Geometry: final body of the model. Coordinates: model frame, mm. A direction names the side the tool comes from. Coordinates: 2 decimals unless noted, no trailing zeros. Order: outer loops, then holes, each group sorted by start corner. A loop starts at its lowest first (then second) coordinate and runs counter-clockwise, first axis right, second up. Notation, with made-up numbers: M -34.5,-10 L 0.5,-10 A37 ccw 0.5,26 Z; hole C 39,41 d10. An arc over 180 degrees is marked long. Use CSV: the item, a comma, the result in double quotes. Start each with the question number.
Q1. Section query A-A, the plane z = -116.5. Output: boundary loops of the cut face in (x, y).
Q2. Access query for faces 1 (the face through (7, 5.5, -150)), 2 (the face through (2, 6, -127.5)), 3 (the face through (2, 4, -142.5)), 4 (the face through (3.5, 6.883, 151.232)). Directions: +Z, -Z, +X, -X, +Y, -Y. A direction counts if a zero-diameter tool reaches every point of the face in a straight line with its end or side. Return the directions, or none.
Q3. First-contact query: P1, Ø5, axis at y = 2, z = 48.5, coming from the +X side; P2, Ø2, axis at y = 2, z = -70.5, coming from the -X side; P3, Ø5, axis at x = 3, z = -82, coming from the +Y side. Flat tips, straight axial feed; report the tip coordinate or a pass-through.
Q4. Mould query, pull axis X, two halves, no side actions, for faces 5 (the face through (2.168, 8.497, -151.486)), 6 (the face through (4, 6, -146)), 7 (the face through (-3.5, 5, -139)), 8 (the face through (7.2, 5.1, 150)). Classes: +X half, -X half, draft (parallel to the pull), parting line (faces both ways), or undercut.
Q5. Ray query, probe 1 along Z at (x, y) = (7.25, 4); probe 2 along Z at (x, y) = (2, 7.7); probe 3 along Z at (x, y) = (2, 1). Return the intervals inside material, ascending.
Autodesk Inventor part; units mm, degrees
ref_plane "YZ Plane" through (0, 0, 0) normal (1, 0, 0) x (0, 1, 0)
ref_plane "XZ Plane" through (0, 0, 0) normal (0, 1, 0) x (-1, 0, 0)
ref_plane "XY Plane" through (0, 0, 0) normal (0, 0, 1) x (1, 0, 0)
sketch "Sketch1" plane through (0, 0, 0) normal (0, 0, 1) x (1, 0, 0)
  line L0 (0, 0) -> (4, 0)
  line L1 (4, 0) -> (4, 4)
  line L2 (4, 4) -> (0, 4)
  line L3 (0, 4) -> (0, 0)
  dimension "d0" = 4
  dimension "d1" = 4
extrude "Extrusion1" add sketch "Sketch1" along normal blind 138.5
sketch "Sketch3" plane through (0, 0, 138.5) normal (0, 0, 1) x (1, 0, 0)
  line L0 (0, 0) -> (4, 0)
  line L1 (-3.5, 0) -> (7.5, 0)
  line L2 (7.5, 0) -> (7.5, 8)
  line L3 (7.5, 8) -> (-3.5, 8)
  line L4 (-3.5, 8) -> (-3.5, 0)
  point P0 (2, 0)
  dimension "d4" = 11
  dimension "d5" = 8
extrude "Extrusion2" add sketch "Sketch3" along normal blind 11.5
sketch "Sketch4" plane through (0, 0, 0) normal (0, -1, 0) x (1, 0, 0)
  line L0 (7.5, 138.5) -> (7.5, 150)
  line L1 (-3.5, 150) -> (7.5, 150)
  line L2 (-1.75, 146) -> (5.75, 146)
  line L3 (5.75, 146) -> (5.75, 142.5)
  line L4 (5.75, 142.5) -> (-1.75, 142.5)
  line L5 (-1.75, 142.5) -> (-1.75, 146)
  point P0 (2, 146)
  point P1 (2, 150)
  point P2 (5.75, 144.25)
  point P3 (7.5, 144.25)
  dimension "d8" = 7.5
  dimension "d9" = 3.5
extrude "Extrusion3" cut sketch "Sketch4" against normal blind 8
sketch "Sketch5" plane through (0, 0, 150) normal (0, 0, 1) x (1, 0, 0)
  circle A0 centre (2, 4) radius 2.1
  point P0 (0, 0)
  dimension "d12" = 4.2
extrude "Extrusion4" cut sketch "Sketch5" against normal up to surface (7.5 mm away)
sketch "Sketch6" plane through (-3.5, 8, 138.5) normal (0, 1, 0) x (1, 0, 0)
  line L0 (11, 0) -> (0, 0)
  line L1 (0, 0) -> (0, -11.5)
  line L2 (11, -11.5) -> (0, -11.5)
  line L3 (11, 0) -> (11, -11.5)
  point P0 (3.5, 138.5)
extrude "Extrusion5" add sketch "Sketch6" along normal blind 1
mirror "Mirror2" about plane through (0, 0, 0) normal (0, 0, 1) of "Extrusion1", "Extrusion5", "Extrusion2", "Extrusion3", "Extrusion4"
sketch "Sketch7" plane through (0, 0, 150) normal (0, 0, 1) x (1, 0, 0)
  line L0 (-3.5, 0) -> (7.5, 0)
  arc A0 (4.0616, 0) -> (-0.0616, 0) centre (2, 4) ccw
  line L1 (0, 0) -> (-0.0616, 0)
  line L2 (-0.0616, 0) -> (4.0616, 0)
  circle A1 centre (2, 4) radius 3.25
  dimension "d17" = 9
  dimension "d18" = 6.5
extrude "Extrusion6" add sketch "Sketch7" along normal blind 2.5
sketch "Sketch8" plane through (-3.5, 8, 138.5) normal (0, -1, 0) x (1, 0, 0)
  line L0 (1.75, 7.5) -> (1.75, 4)
  line L1 (1.75, 4) -> (9.25, 4)
  line L2 (9.25, 4) -> (9.25, 7.5)
  line L3 (9.25, 7.5) -> (1.75, 7.5)
  point P0 (3.5, -138.5)
mirror "Mirror3" about plane through (0, 0, 0) normal (0, 0, 1) of "Extrusion6"
sketch "Sketch10" plane through (-3.5, 9, -138.5) normal (0, 1, 0) x (1, 0, 0)
  line L0 (0, 0) -> (11, 0)
  line L1 (11, 0) -> (11, -9)
  line L2 (11, -9) -> (0, -9)
  line L3 (0, -9) -> (0, 0)
  point P0 (3.5, -138.5)
  dimension "d21" = 9
extrude "Extrusion7" add sketch "Sketch10" against normal up to surface (9 mm away)
sketch "Sketch11" plane through (-3.5, 9, -150) normal (0, 1, 0) x (1, 0, 0)
  line L0 (11, -20.5) -> (0, -20.5)
  circle A0 centre (5.5, -15) radius 2.1
  point P0 (3.5, -150)
  dimension "d24" = 4.2
  dimension "d25" = 5.5
extrude "Extrusion8" cut sketch "Sketch11" against normal blind 11
sketch "Sketch12" plane through (-3.5, 0, -150) normal (-1, 0, 0) x (0, 0, 1)
  line L0 (20.5, 9) -> (20.5, 0)
  line L1 (18.75, 6.25) -> (11.25, 6.25)
  line L2 (11.25, 6.25) -> (11.25, 2.75)
  line L3 (11.25, 2.75) -> (18.75, 2.75)
  line L4 (18.75, 2.75) -> (18.75, 6.25)
  point P0 (150, 0)
  point P1 (18.75, 4.5)
  point P2 (20.5, 4.5)
  dimension "d28" = 7.5
  dimension "d29" = 3.5
  dimension "d30" = 1.75
extrude "Extrusion9" cut sketch "Sketch12" against normal blind 11
fillet "Fillet3" radius 0.5 1 edges at (2, 8.5, -150)
sketch "Sketch14" plane through (-3.5, 9, -129.5) normal (0, 0, 1) x (1, 0, 0)
  line L0 (7.5, -9) -> (7.5, -5)
  line L1 (7.5, -9) -> (11, -9)
  line L2 (11, 0) -> (11, -9)
  line L3 (11, 0) -> (0, 0)
  line L4 (0, 0) -> (0, -9)
  line L5 (0, -9) -> (3.5, -9)
  line L6 (3.5, -5) -> (3.5, -9)
  line L7 (7.5, -5) -> (3.5, -5)
extrude "Extrusion10" add sketch "Sketch14" along normal blind 2
fillet "Fillet4" radius 1.5 3 edges at (4, 2, -127.5) (2, 4, -127.5) (0, 2, -127.5)
mirror "Mirror5" about plane through (0, 0, 0) normal (0, 0, 1) of "Extrusion7", "Extrusion8", "Extrusion9", "Extrusion10"
fillet "Fillet5" radius 1.5 3 edges at (0, 2, 127.5) (2, 4, 127.5) (4, 2, 127.5)
fillet "Fillet6" radius 0.5 1 edges at (2, 8.5, 150)
properties part number "Axle300mm"
Responses:
1,outline,"M 0,0 L 4,0 L 4,4 L 0,4 Z"
2,face 1,"-Z, +X"
2,face 2,"+Y"
2,face 3,"-Y"
2,face 4,"+Z"
3,P1,"stops at x = 4"
3,P2,"stops at x = 0"
3,P3,"stops at y = 4"
4,face 5,"parting line"
4,face 6,"undercut"
4,face 7,"-X half"
4,face 8,"draft"
5,probe 1,"z = -150 to -138.75, -131.25 to -127.5, 127.5 to 131.25, 138.75 to 150"
5,probe 2,"z = -152.5 to -146, -142.5 to -137.1, -132.9 to -127.5, 127.5 to 132.9, 137.1 to 142.5, 146 to 152.5"
5,probe 3,"z = -150 to -146, -142.5 to -137.1, -132.9 to 132.9, 137.1 to 142.5, 146 to 150"
